from build123d import *

# Parameters (mm, degrees)
EXTRUDE_2_DEPTH          = 2
CUT_EXTRUDE_5_DEPTH      = 42.806183605
PATTERN_START            = -2
PATTERN_LINEAR_6_DEPTH   = 2
PATTERN_CIRCULAR_2_COUNT = 5


# Read off the part's stored shape, not the designer's step: Линейный массив6
with BuildPart() as part:
    # Эскиз6 → Бобышка-Вытянуть2 (new body)
    with BuildSketch(Plane.XY):
        with BuildLine():
            Line((0, 0), (-21.160269083, 29.124611797))
            ThreePointArc((-21.160269083, 29.124611797), (0, 36), (21.160269083, 29.124611797))
            Line((21.160269083, 29.124611797), (0, 0))
        make_face()
    extrude_2 = extrude(amount=-EXTRUDE_2_DEPTH)

    # Эскиз8 → Вырез-Вытянуть5 (cut, through all)
    with BuildSketch(Plane.XY):
        with BuildLine():
            ThreePointArc((2.763082425, 8.728809248), (0, 9.15569415), (-2.763082425, 8.728809248))
            ThreePointArc((-2.763082425, 8.728809248), (-3.577565566, 7.15985507), (-2.008611388, 6.345371929))
            ThreePointArc((-2.008611388, 6.345371929), (0, 6.65569415), (2.008611388, 6.345371929))
            ThreePointArc((2.008611388, 6.345371929), (3.577565566, 7.15985507), (2.763082425, 8.728809248))
        make_face()
    cut_extrude_5 = extrude(amount=-CUT_EXTRUDE_5_DEPTH, mode=Mode.SUBTRACT)

    # Линейный массив6 outline → Линейный массив6 (cut)
    with BuildSketch(Plane.XY.offset(PATTERN_START)):
        with BuildLine():
            ThreePointArc((-10.584064165, 18.586121936), (0, 21.388462845), (10.584064165, 18.586121936))
            ThreePointArc((10.584064165, 18.586121936), (12.288849258, 19.053783979), (11.821187216, 20.758569072))
            ThreePointArc((11.821187216, 20.758569072), (0, 23.888462845), (-11.821187216, 20.758569072))
            ThreePointArc((-11.821187216, 20.758569072), (-12.288849258, 19.053783979), (-10.584064165, 18.586121936))
        make_face()
        with BuildLine():
            ThreePointArc((-7.679367639, 14.522246343), (0, 16.42766953), (7.679367639, 14.522246343))
            ThreePointArc((7.679367639, 14.522246343), (9.368713619, 15.042928742), (8.84803122, 16.732274722))
            ThreePointArc((8.84803122, 16.732274722), (0, 18.92766953), (-8.84803122, 16.732274722))
            ThreePointArc((-8.84803122, 16.732274722), (-9.368713619, 15.042928742), (-7.679367639, 14.522246343))
        make_face()
        with BuildLine():
            ThreePointArc((-16.425471774, 26.69787158), (0, 31.346012026), (16.425471774, 26.69787158))
            ThreePointArc((16.425471774, 26.69787158), (18.145122081, 27.107509008), (17.735484653, 28.827159315))
            ThreePointArc((17.735484653, 28.827159315), (0, 33.846012026), (-17.735484653, 28.827159315))
            ThreePointArc((-17.735484653, 28.827159315), (-18.145122081, 27.107509008), (-16.425471774, 26.69787158))
        make_face()
        with BuildLine():
            ThreePointArc((-13.501393974, 22.643792845), (0, 26.363402543), (13.501393974, 22.643792845))
            ThreePointArc((13.501393974, 22.643792845), (15.215189583, 23.077272498), (14.78170993, 24.791068107))
            ThreePointArc((14.78170993, 24.791068107), (0, 28.863402543), (-14.78170993, 24.791068107))
            ThreePointArc((-14.78170993, 24.791068107), (-15.215189583, 23.077272498), (-13.501393974, 22.643792845))
        make_face()
        with BuildLine():
            ThreePointArc((-4.802636201, 10.446449807), (0, 11.497548784), (4.802636201, 10.446449807))
            ThreePointArc((4.802636201, 10.446449807), (6.460498921, 11.060038594), (5.846910135, 12.717901314))
            ThreePointArc((5.846910135, 12.717901314), (0, 13.997548784), (-5.846910135, 12.717901314))
            ThreePointArc((-5.846910135, 12.717901314), (-6.460498921, 11.060038594), (-4.802636201, 10.446449807))
        make_face()
    pattern_linear_6 = extrude(amount=PATTERN_LINEAR_6_DEPTH, mode=Mode.SUBTRACT)

    # Круговой массив2: Бобышка-Вытянуть2, Вырез-Вытянуть5, Линейный массив6 ×5 about axis
    pattern_circular_2_axis = Axis((0, 0, 0), (0, 0, 1))
    add([extrude_2.rotate(pattern_circular_2_axis, i * 360 / PATTERN_CIRCULAR_2_COUNT) for i in range(1, PATTERN_CIRCULAR_2_COUNT)])
    add([cut_extrude_5.rotate(pattern_circular_2_axis, i * 360 / PATTERN_CIRCULAR_2_COUNT) for i in range(1, PATTERN_CIRCULAR_2_COUNT)], mode=Mode.SUBTRACT)
    add([pattern_linear_6.rotate(pattern_circular_2_axis, i * 360 / PATTERN_CIRCULAR_2_COUNT) for i in range(1, PATTERN_CIRCULAR_2_COUNT)], mode=Mode.SUBTRACT)


solid = part.part
Part model, mm, in its own coordinate system. Round coordinates to 2 decimals unless told otherwise and drop trailing zeros. Write each loop counter-clockwise with the first axis right and the second up, starting at its lowest first coordinate (ties: lowest second). Pieces come first, ordered by that corner, then holes. Notation, with made-up numbers: M -16.5,88.5 L 39.5,88.5 A32 cw 39.5,114.5 Z; hole C 5,6 d10. An arc over 180 degrees is marked long. Return JSON: item names as keys, results as strings. Group by question number.
(1) Drill centre lines: probe 1 along Y at (x, z) = (-22, -1.4); probe 2 along Y at (x, z) = (-24, -0.25). Where is each one in solid material? Low to high.
(2) Saw through at A-A on y = -27.5. Write the cut outline in (x, z), then the cut area to 3 significant figures.
(3) Saw through at B-B on z = -0.6. Count the separate pieces of the cut face and the enclosed holes in it, then the cut area to 3 significant figures.
Returned:
{
 "1": {"probe 1": "-28.5 to -25.72, -22.33 to -18.68, -14.53 to -5.81, 9.31 to 14.53, 18.68 to 22.33, 25.72 to 28.5", "probe 2": "-26.83 to -23.87, -20.16 to -16.03, -10.91 to 10.91, 16.03 to 20.16, 23.87 to 26.83"},
 "2": {"outline": "M -23.23,-2 L -19.73,-2 L -19.73,0 L -23.23,0 Z; M -15.04,-2 L -8.77,-2 L -8.77,0 L -15.04,0 Z; M -1.25,-2 L 1.25,-2 L 1.25,0 L -1.25,0 Z; M 8.77,-2 L 15.04,-2 L 15.04,0 L 8.77,0 Z; M 19.73,-2 L 23.23,-2 L 23.23,0 L 19.73,0 Z", "area": "44.1 mm²"},
 "3": {"separate pieces": "1", "enclosed holes": "30", "area": "2,400 mm²"}
}
